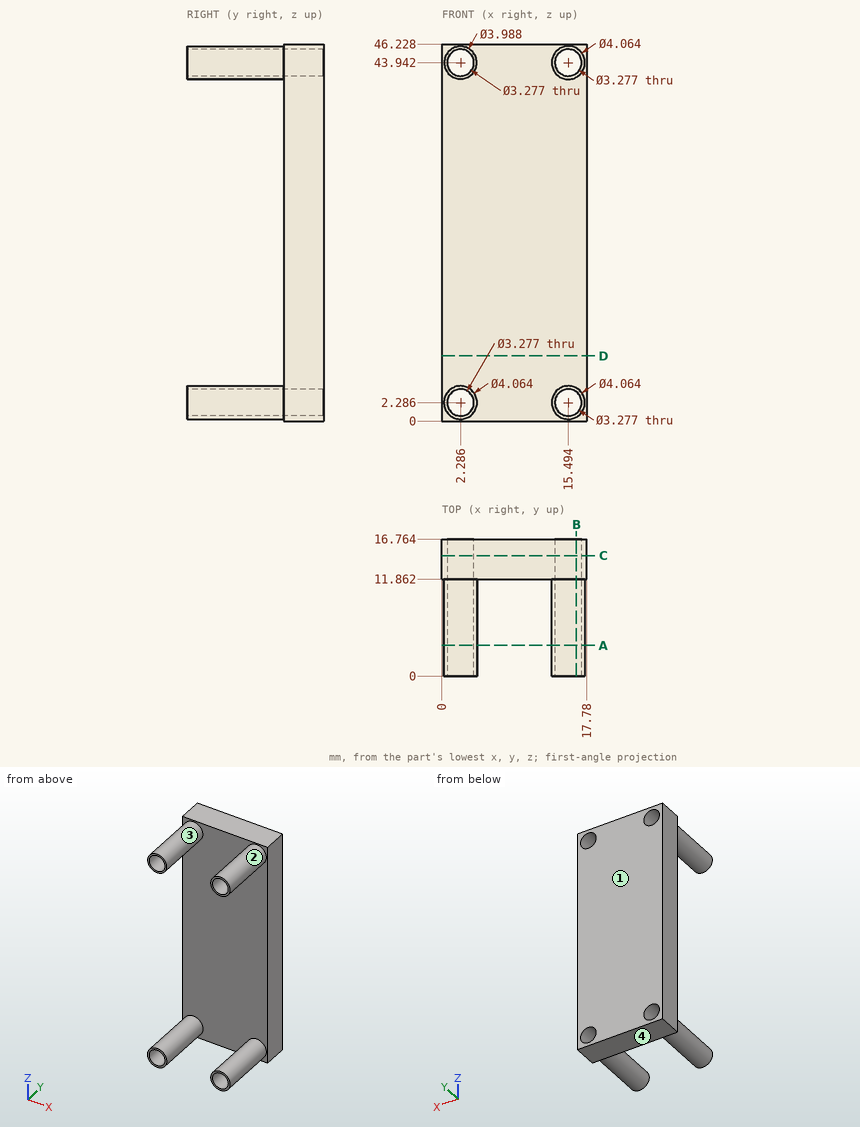
The figure shows three views and two pictorial views of one solid part (mm, origin at its lowest corner). Answer the questions. A direction names the side the tool comes from. Coordinates: 2 decimals unless noted, no trailing zeros. Order: outer loops, then holes, each group sorted by start corner. A loop starts at its lowest first (then second) coordinate and runs counter-clockwise, first axis right, second up. Notation, with made-up numbers: (62.5, 53) - (77.5, 53) arc R12 cw to (77.5, 75) - close; hole circle Ø8 at (-34, 8.5). An arc over 180 degrees is marked (long way). Answer as a JSON object with one key per item and string values.
1. A tool of negligible diameter and unlimited length cuts with its end or side. For the marked faces 3 and 4, from which of +Z, -Z, +X, -X, +Y, -Y can it reach the whole face along a straight path? Write none if from no direction.
Output values:
{"face 3": "-Y", "face 4": "-Z, +X, -X, +Y, -Y"}
2. Consider line 1 (Z direction, x = 15.5, y = 15.25) (1 decimal); line 2 (Z direction, x = 15, y = 10.75) (1 decimal); line 3 (X direction, y = 13, z = 44.5) (1 decimal). Determine where each line is inside the solid, lowest interval first.
Output values:
{"line 1": "z = 0 to 0.6, 3.9 to 42.3, 45.6 to 46.2", "line 2": "z = 0.3 to 0.7, 3.8 to 4.3, 42 to 42.4, 45.5 to 45.9", "line 3": "x = 0 to 0.7, 3.8 to 14, 17 to 17.8"}
3. The mould has two halves that part along X. Classify the marked faces 1 and 2: +X half, -X half, draft (parallel to the pull), parting line (faces both ways), or undercut.
Output values:
{"face 1": "draft", "face 2": "undercut"}
4. Each of these flat-tipped pins is pushed along its axis until it touches: P1, Ø2, axis at x = 2, y = 6, coming from the -Z side; P2, Ø5.5, axis at x = 12.5, z = 15.5, coming from the -Y side. Where does it stop, or does it pass through?
Output values:
{"P1": "stops at z = 0.25", "P2": "stops at y = 11.86"}
5. Find section B-B on x = 16.5. Determine the outline of the cut face in (y, z) (1 decimal).
Output values:
{"outline": "(0, 0.5) - (11.9, 0.5) - (11.9, 0) - (16.8, 0) - (16.8, 1) - (0, 1) - close; (0, 3.6) - (16.8, 3.6) - (16.8, 42.6) - (0, 42.6) - (0, 42.2) - (11.9, 42.2) - (11.9, 4.1) - (0, 4.1) - close; (0, 45.2) - (16.8, 45.2) - (16.8, 46.2) - (11.9, 46.2) - (11.9, 45.7) - (0, 45.7) - close"}
6. Find section A-A on y = 3.75. Determine the outline of the cut face in (x, z) (1 decimal).
Output values:
{"outline": "circle Ø4.1 at (2.3, 2.3); circle Ø4 at (2.3, 43.9); circle Ø4.1 at (15.5, 2.3); circle Ø4.1 at (15.5, 43.9); hole circle Ø3.3 at (2.3, 2.3); hole circle Ø3.3 at (2.3, 43.9); hole circle Ø3.3 at (15.5, 2.3); hole circle Ø3.3 at (15.5, 43.9)"}
7. Find section D-D on z = 8. Determine the outline of the cut face in (x, y).
Output values:
{"outline": "(0, 11.86) - (17.78, 11.86) - (17.78, 16.76) - (0, 16.76) - close"}
8. Find section C-C on y = 14.75. Determine the outline of the cut face in (x, z) (1 decimal).
Output values:
{"outline": "(0, 0) - (17.8, 0) - (17.8, 46.2) - (0, 46.2) - close; hole circle Ø3.3 at (2.3, 2.3); hole circle Ø3.3 at (2.3, 43.9); hole circle Ø3.3 at (15.5, 2.3); hole circle Ø3.3 at (15.5, 43.9)"}
